```python
from build123d import *

# Parameters (mm, degrees)
SKETCH1_W           = 52
SKETCH1_H           = 24
SKETCH1_R           = 8.25
BOSS_EXTRUDE1_DEPTH = 12
SKETCH2_R           = 1
CUT_EXTRUDE1_DEPTH  = 32.048349393
SKETCH3_R           = 1.75
CUT_EXTRUDE2_DEPTH  = 1
CUT_EXTRUDE3_DEPTH  = 5
FILLET2_R           = 0.5
SKETCH6_W           = 10
SKETCH6_H           = 10
SKETCH6_R           = 2
BOSS_EXTRUDE2_DEPTH = 5
FILLET3_R           = 4.6
FILLET4_R           = 3
SKETCH9_R           = 1.75
BOSS_EXTRUDE3_DEPTH = 12
SKETCH10_W          = 13.41545795
SKETCH10_H          = 24
SKETCH10_W_2        = 15.564044944
CUT_EXTRUDE4_DEPTH  = 39.587562763
FILLET5_R           = 3


with BuildPart() as part:
    # Sketch1 → Boss-Extrude1 (new body)
    with BuildSketch(Plane(origin=(0, 0, 0), x_dir=(1, 0, 0), z_dir=(0, 1, 0))):
        Rectangle(SKETCH1_W, SKETCH1_H)
        with Locations(Location((12.75, 0, 0), (0, 0, 270))):
            Circle(SKETCH1_R, mode=Mode.SUBTRACT)
        with Locations(Location((-12.75, 0, 0), (0, 0, 270))):
            Circle(SKETCH1_R, mode=Mode.SUBTRACT)
    extrude(amount=BOSS_EXTRUDE1_DEPTH)

    # Sketch2 → Cut-Extrude1 (cut, through all)
    with BuildSketch(Plane(origin=(0, 12, 0), x_dir=(1, 0, 0), z_dir=(0, 1, 0))):
        with Locations(Location((-21.35, 8.85, 0), (0, 0, 270))):
            Circle(SKETCH2_R)
        with Locations(Location((21.35, 8.85, 0), (0, 0, 270))):
            Circle(SKETCH2_R)
        with Locations(Location((21.35, -8.85, 0), (0, 0, 270))):
            Circle(SKETCH2_R)
        with Locations(Location((-21.35, -8.85, 0), (0, 0, 270))):
            Circle(SKETCH2_R)
    extrude(amount=-CUT_EXTRUDE1_DEPTH, mode=Mode.SUBTRACT)

    # Sketch3 → Cut-Extrude2 (cut)
    with BuildSketch(Plane(origin=(0, 12, 0), x_dir=(1, 0, 0), z_dir=(0, 1, 0))):
        with Locations(Location((-21.35, 8.85, 0), (0, 0, 270))):
            Circle(SKETCH3_R)
        with Locations(Location((21.35, 8.85, 0), (0, 0, 270))):
            Circle(SKETCH3_R)
        with Locations(Location((21.35, -8.85, 0), (0, 0, 270))):
            Circle(SKETCH3_R)
        with Locations(Location((-21.35, -8.85, 0), (0, 0, 270))):
            Circle(SKETCH3_R)
    extrude(amount=-CUT_EXTRUDE2_DEPTH, mode=Mode.SUBTRACT)

    # Sketch4 → Cut-Extrude3 (cut)
    with BuildSketch(Plane.XZ):
        Polygon((-6, -5), (-6, -12), (6, -12), (6, -5), (0, -5), align=None)
    extrude(amount=-CUT_EXTRUDE3_DEPTH, mode=Mode.SUBTRACT)

    # Fillet2
    fillet2_edges = [part.edges().sort_by_distance(p)[0] for p in [
        (0, 5, -12),
        (6, 2.5, -12),
        (-6, 2.5, -12),
        (-6, 2.5, -5),
        (6, 5, -8.5),
        (6, 2.5, -5),
        (-6, 5, -8.5),
        (0, 5, -5),
    ]]
    fillet(fillet2_edges, radius=FILLET2_R)

    # Sketch6 → Boss-Extrude2 (add)
    # profile 1 of 2: a face of its own
    with BuildSketch(Plane(origin=(0, 12, 0), x_dir=(1, 0, 0), z_dir=(0, 1, 0))):
        with Locations((-31, 0)):
            Rectangle(SKETCH6_W, SKETCH6_H)
        with Locations(Location((-31, 0, 0), (0, 0, 270))):
            Circle(SKETCH6_R, mode=Mode.SUBTRACT)
    # profile 2 of 2: a face of its own
    with BuildSketch(Plane(origin=(0, 12, 0), x_dir=(1, 0, 0), z_dir=(0, 1, 0))):
        with Locations((31, 0)):
            Rectangle(SKETCH6_W, SKETCH6_H)
        with Locations(Location((31, 0, 0), (0, 0, 90))):
            Circle(SKETCH6_R, mode=Mode.SUBTRACT)
    extrude(amount=-BOSS_EXTRUDE2_DEPTH)

    # Fillet3
    fillet3_edges = [part.edges().sort_by_distance(p)[0] for p in [
        (-26, 9.5, -5),
        (-26, 9.5, 5),
        (26, 9.5, -5),
        (26, 9.5, 5),
    ]]
    fillet(fillet3_edges, radius=FILLET3_R)

    # Fillet4
    fillet4_edges = [part.edges().sort_by_distance(p)[0] for p in [
        (-36, 9.5, 5),
        (-36, 9.5, -5),
        (36, 9.5, -5),
        (36, 9.5, 5),
    ]]
    fillet(fillet4_edges, radius=FILLET4_R)

    # Sketch9 → Boss-Extrude3 (add)
    with BuildSketch(Plane(origin=(0, 12, 0), x_dir=(1, 0, 0), z_dir=(0, 1, 0))):
        with Locations((-21.35, -8.85)):
            Circle(SKETCH9_R)
        with Locations((21.35, -8.85)):
            Circle(SKETCH9_R)
        with Locations((21.35, 8.85)):
            Circle(SKETCH9_R)
        with Locations((-21.35, 8.85)):
            Circle(SKETCH9_R)
    extrude(amount=-BOSS_EXTRUDE3_DEPTH)

    # Sketch10 → Cut-Extrude4 (cut, through all)
    with BuildSketch(Plane.XZ.offset(-7)):
        with Locations((-32.707728975, 0)):
            Rectangle(SKETCH10_W, SKETCH10_H)
        with Locations((33.782022472, 0)):
            Rectangle(SKETCH10_W_2, SKETCH10_H)
    extrude(amount=-CUT_EXTRUDE4_DEPTH, mode=Mode.SUBTRACT)

    # Fillet5
    # the kernel refuses this fillet: 3 mm, written as the material it takes off along each edge
    with BuildSketch(Plane(origin=(-26, 12, -19.5), x_dir=(1, 0, 0), z_dir=(0, 0, 1)), Plane(origin=(26, 12, 19.5), x_dir=(-1, 0, 0), z_dir=(0, 0, -1))) as fillet5_piece_1:
        with BuildLine():
            CenterArc((FILLET5_R, -FILLET5_R), FILLET5_R, 90, 90)
            Line((0, -FILLET5_R), (0, 0))
            Line((0, 0), (FILLET5_R, 0))
        make_face()
    extrude(amount=39, mode=Mode.SUBTRACT)
    with BuildSketch(Plane(origin=(12.75, 12, 0), x_dir=(0, 0, 1), z_dir=(-1, 0, 0))) as fillet5_piece_2:
        with BuildLine():
            CenterArc((8.25 + FILLET5_R, -FILLET5_R), FILLET5_R, 90, 90)
            Line((8.25, -FILLET5_R), (8.25, 0))
            Line((8.25, 0), (8.25 + FILLET5_R, 0))
        make_face()
    revolve(axis=Axis((12.75, 12, 0), (0, 1, 0)), mode=Mode.SUBTRACT)
    with BuildSketch(Plane(origin=(-12.75, 12, 0), x_dir=(0, 0, 1), z_dir=(-1, 0, 0))) as fillet5_piece_3:
        with BuildLine():
            CenterArc((8.25 + FILLET5_R, -FILLET5_R), FILLET5_R, 90, 90)
            Line((8.25, -FILLET5_R), (8.25, 0))
            Line((8.25, 0), (8.25 + FILLET5_R, 0))
        make_face()
    revolve(axis=Axis((-12.75, 12, 0), (0, 1, 0)), mode=Mode.SUBTRACT)


solid = part.part
```
Work out the finished part from the listing and answer in its coordinate system (mm). A direction names the side the tool comes from. Give positions to 0.01 mm unless a question says otherwise; leave off trailing zeros. Order: outer loops, then holes, each group sorted by start corner. A loop starts at its lowest first (then second) coordinate and runs counter-clockwise, first axis right, second up. Notation, with made-up numbers: (34.5, -11) -> (89.5, -11) arc R27 ccw to (89.5, 11) -> close; hole circle Ø3 at (-15.5, 88). An arc over 180 degrees is marked (long way). Answer as CSV lines item,"result". Start each with the question number.
(1) Each of these flat-tipped pins is pushed along its axis until it touches: pin 1 Ø8 at (x, z) = (-6.5, 3) entering from -Y; pin 2 Ø13 at (x, z) = (-12.75, 0) entering from +Y; pin 3 Ø3.5 at (x, y) = (1.5, 3) entering from -Z; pin 4 Ø1.5 at (x, z) = (7, -8.5) entering from +Y. Where does it stop, or does it pass through?
(2) Section B-B, the plane y = 7 is taken. Write down the section's boundary in (x, z), plus the area to 3 significant figures.
(3) Section C-C, the plane z = 0 is taken. Write down the section's boundary in (x, y), plus the area to 3 significant figures.
(4) Consider line 1 along X through (y, z) = (6, 0); line 2 along X through (y, z) = (3.75, -1); line 3 along Z through (x, y) = (20, 2). Determine where each line is inside the solid, lowest interval first.
(5) Section D-D, the plane x = -1 is taken. Write down the section's boundary in (y, z), plus the area to 3 significant figures.
(6) Which of the six approach directions +Z, -Z, +X, -X, +Y, -Y give full straight-line access (tool end or side, diameter ignored) to faces 1 (the flat face through (0, 2, -5)), 2 (the flat face through (0, 6, -12))?
(7) For a pull along X with two mould halves and no side action, classify faces 3 (the flat face through (-26, 4, 0)), 4 (the flat face through (-6, 2, -8)), 5 (the flat face through (0, 0, 0)) as released by +X, released by -X, zero draft, split by the parting line, or undercut.
(8) Section A-A, the plane x = -12.75 is taken. Write down the section's boundary in (y, z), plus the area to 3 significant figures.
Entries:
1,pin 1,"y = 0"
1,pin 2,"through"
1,pin 3,"z = -5.07"
1,pin 4,"y = 11.99"
2,outline,"(-26, -12) -> (26, -12) -> (26, 12) -> (-26, 12) -> close; hole circle Ø16.5 at (-12.75, 0); hole circle Ø16.5 at (12.75, 0)"
2,area,"820 mm²"
3,outline,"(-26, 0) -> (-21, 0) -> (-21, 9) arc R3 ccw to (-23.5, 11.96) arc R3 ccw to (-26, 9) -> close; (-4.5, 0) -> (4.5, 0) -> (4.5, 9) arc R3 ccw to (1.5, 12) -> (-1.5, 12) arc R3 ccw to (-4.5, 9) -> close; (21, 0) -> (26, 0) -> (26, 9) arc R3 ccw to (23.5, 11.96) arc R3 ccw to (21, 9) -> close"
3,area,"216 mm²"
4,line 1,"-26 to -21, -4.5 to 4.5, 21 to 26"
4,line 2,"-26 to -20.94, -4.56 to 4.56, 20.94 to 26"
4,line 3,"-12 to -3.94, 3.94 to 12"
5,outline,"(0, -5) -> (4.5, -5) arc R0.5 cw to (5, -5.5) -> (5, -11.5) arc R0.5 ccw to (5.5, -12) -> (12, -12) -> (12, 12) -> (0, 12) -> close"
5,area,"253 mm²"
6,face 1,"-Z, -Y"
6,face 2,"-Z, +X, -X, +Y, -Y"
7,face 3,"released by -X"
7,face 4,"undercut"
7,face 5,"zero draft"
8,outline,"(0, -12) -> (12, -12) -> (12, -11.25) arc R3 ccw to (9, -8.25) -> (0, -8.25) -> close; (0, 8.25) -> (9, 8.25) arc R3 ccw to (12, 11.25) -> (12, 12) -> (0, 12) -> close"
8,area,"86.1 mm²"
